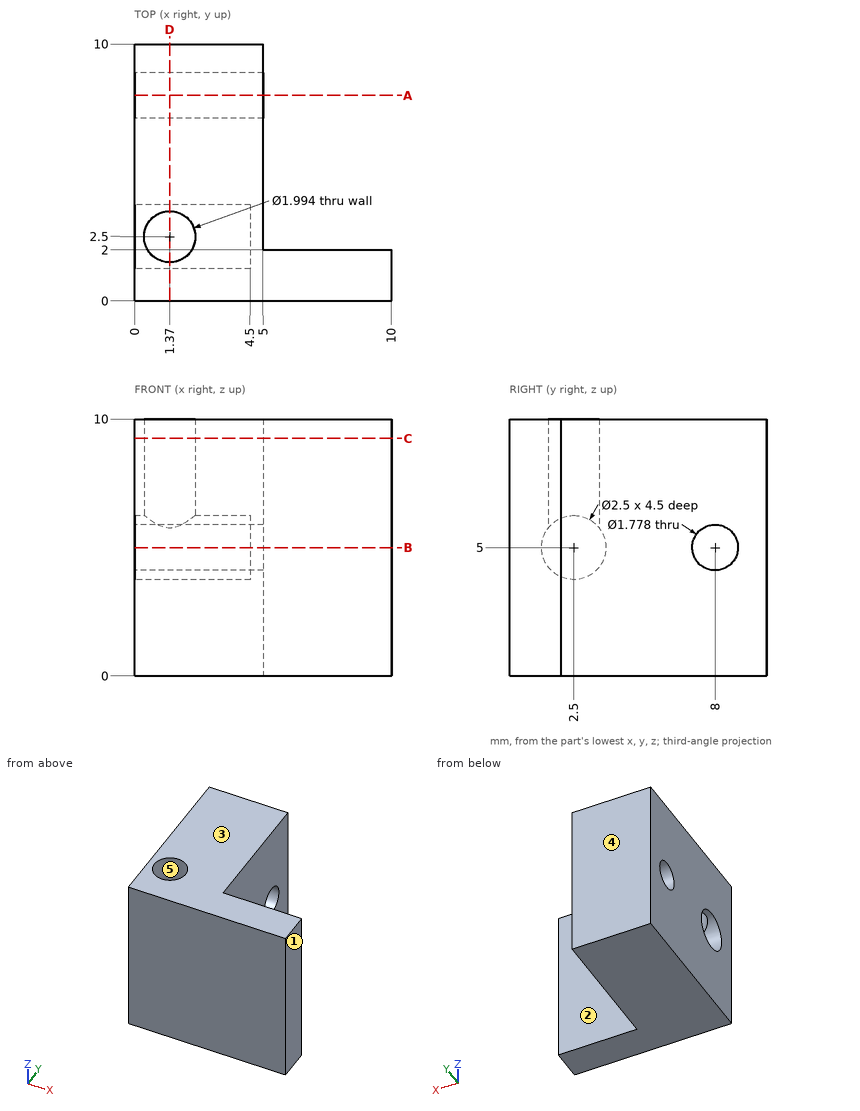
Geometry: see drawing. Coordinates: mm, zero at the bounding-box minimum. A direction names the side the tool comes from. Coordinates: 2 decimals unless noted, no trailing zeros. Loops run counter-clockwise (first coordinate to the right, second up) from the corner with the lowest first, then second, coordinate; pieces in that order, holes last. Notation, with made-up numbers: M -16,26 L 1,26 A12 ccw 1,42 Z; hole C 50.5,20 d6. An arc over 180 degrees is marked long. Answer in a Markdown table with one row per item.
Q1. Draft query along Y for the marked faces 3, 4 and 5. Return one class per face: pulls with the +Y half, pulls with the -Y half, needs draft (parallel to the pull), parting line crosses it, or undercut.
Answers below:
| item | result |
|---|---|
| face 3 | needs draft |
| face 4 | pulls with the +Y half |
| face 5 | undercut |
Q2. Section C-C on z = 9.25. Return the cut outline in (x, y), plus the area to 3 significant figures.
Answers below:
| item | result |
|---|---|
| outline | M 0,0 L 10,0 L 10,2 L 5,2 L 5,10 L 0,10 Z; hole C 1.37,2.5 d1.99 |
| area | 56.9 mm^2 |
Q3. Section A-A on y = 8. Return the cut outline in (x, z), plus the area to 3 significant figures.
Answers below:
| item | result |
|---|---|
| outline | M 0,0 L 5,0 L 5,4.11 L 0,4.11 Z; M 0,5.89 L 5,5.89 L 5,10 L 0,10 Z |
| area | 41.1 mm^2 |
Q4. Section B-B on z = 5. Return the cut outline in (x, y).
Answers below:
| item | result |
|---|---|
| outline | M 0,0 L 10,0 L 10,2 L 5,2 L 5,7.11 L 0,7.11 L 0,3.75 L 4.5,3.75 L 4.5,1.25 L 0,1.25 Z; M 0,8.89 L 5,8.89 L 5,10 L 0,10 Z |
Q5. Section D-D on x = 1.37. Return the cut outline in (y, z).
Answers below:
| item | result |
|---|---|
| outline | M 0,0 L 10,0 L 10,10 L 3.5,10 L 3.5,5.75 A1.25 cw long 1.5,5.75 L 1.5,10 L 0,10 Z; hole C 8,5 d1.78 |
Q6. Ray query, probe 1 along Y at (x, z) = (2.6, 5); probe 2 along Y at (x, z) = (1.37, 8.4); probe 3 along X at (y, z) = (4.5, 6.5). Return the intervals inside material, ascending. Write a range as from..to.
Answers below:
| item | result |
|---|---|
| probe 1 | y = 0..1.25, 3.75..7.11, 8.89..10 |
| probe 2 | y = 0..1.5, 3.5..10 |
| probe 3 | x = 0..5 |
Q7. First-contact query: pin 1 (2 mm diameter, centred on y = 8, z = 5, fed in from +X); pin 2 (6 mm diameter, centred on y = 3, z = 4, fed in from +X); pin 3 (0.8 mm diameter, centred on y = 3, z = 5.5, fed in from -X); pin 4 (2.5 mm diameter, centred on x = 6.5, z = 2.5, fed in from +Y). Flat tips, straight axial feed; report the tip coordinate or a pass-through.
Answers below:
| item | result |
|---|---|
| pin 1 | stops at x = 5 |
| pin 2 | stops at x = 10 |
| pin 3 | stops at x = 4.5 |
| pin 4 | stops at y = 2 |
Q8. Set-up query: the marked faces 1 and 2. Return all of +Z, -Z, +X, -X, +Y, -Y with unobstructed straight access to the full face (end or side cutting, diameter ignored); none if empty.
Answers below:
| item | result |
|---|---|
| face 1 | +Z, -Z, +X, +Y, -Y |
| face 2 | +Z, -Z, +X, +Y |
